Job drawing, mm, ordinate dimensions from the low corner. One solid piece. Round coordinates to 2 decimals unless told otherwise and drop trailing zeros. Loops run counter-clockwise (first coordinate to the right, second up) from the corner with the lowest first, then second, coordinate; pieces in that order, holes last. Notation, with made-up numbers: M 60,-31.5 L 92,-31.5 A30 ccw 92,-6.5 Z; hole C 69,16 d10. An arc over 180 degrees is marked long. Use a Markdown table: item, result. Add a question column.
(1) Band-saw the part on A-A, the plane x = 25.4. Write the cut outline in (y, z) (1 decimal).
(2) Wall check: L1, parallel to X at y = 25.4, z = 0.35; L2, parallel to X at y = 28, z = 3.4. Give the ranges that are in metal, low to high.
(3) Flat gauge pin, fed straight in: P1, Ø8, axis at x = 25.4, y = 25.4, coming from the +Z side. Where does the tip first touch, or does it go through?
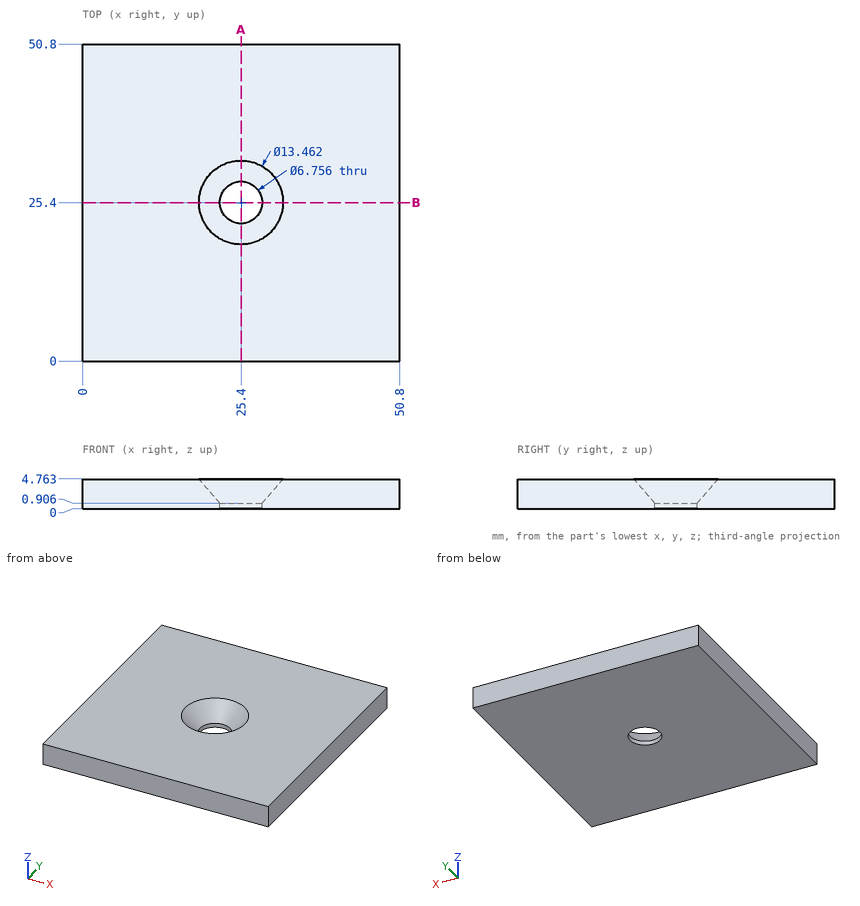
Return value:
| question | item | result |
|---|---|---|
| 1 | outline | M 0,0 L 22,0 L 22,0.9 L 18.7,4.8 L 0,4.8 Z; M 28.8,0 L 50.8,0 L 50.8,4.8 L 32.1,4.8 L 28.8,0.9 Z |
| 2 | L1 | 0 to 22.02, 28.78 to 50.8 |
| 2 | L2 | 0 to 20.5, 30.3 to 50.8 |
| 3 | P1 | z = 1.62 |
